Can you work these out from the model? Positions are in its coordinate system, mm. Coordinates: 2 decimals unless noted, no trailing zeros. Put each result on its own line as item: value. Start each with the question number.
from build123d import *

# Parameters (mm, degrees)
ESQUISSE1_W             = 149
ESQUISSE1_H             = 10
BOSS_EXTRU_1_DEPTH      = 3
ESQUISSE2_R             = 1.005
ESQUISSE2_W             = 5
ESQUISSE2_H             = 3
ENL_V_MAT_EXTRU_1_DEPTH = 150.365323954


with BuildPart() as part:
    # Esquisse1 → Boss.-Extru.1 (new body)
    with BuildSketch(Plane.XY):
        with Locations((74.5, 5)):
            Rectangle(ESQUISSE1_W, ESQUISSE1_H)
    extrude(amount=BOSS_EXTRU_1_DEPTH)

    # Esquisse2 → Enlèv. mat.-Extru.1 (cut, through all)
    with BuildSketch(Plane(origin=(0, 0, 0), x_dir=(-1, 0, 0), z_dir=(0, 0, -1))):
        with Locations((-3, 3)):
            Circle(ESQUISSE2_R)
        with Locations((-146, 3)):
            Circle(ESQUISSE2_R)
        with Locations((-136.5, 6.5)):
            Rectangle(ESQUISSE2_W, ESQUISSE2_H)
        with Locations((-126.5, 6.5)):
            Rectangle(ESQUISSE2_W, ESQUISSE2_H)
        with Locations((-116.5, 6.5)):
            Rectangle(ESQUISSE2_W, ESQUISSE2_H)
        with Locations((-106.5, 6.5)):
            Rectangle(ESQUISSE2_W, ESQUISSE2_H)
        with Locations((-96.5, 6.5)):
            Rectangle(ESQUISSE2_W, ESQUISSE2_H)
        with Locations((-86.5, 6.5)):
            Rectangle(ESQUISSE2_W, ESQUISSE2_H)
        with Locations((-76.5, 6.5)):
            Rectangle(ESQUISSE2_W, ESQUISSE2_H)
        with Locations((-66.5, 6.5)):
            Rectangle(ESQUISSE2_W, ESQUISSE2_H)
        with Locations((-56.5, 6.5)):
            Rectangle(ESQUISSE2_W, ESQUISSE2_H)
        with Locations((-46.5, 6.5)):
            Rectangle(ESQUISSE2_W, ESQUISSE2_H)
        with Locations((-36.5, 6.5)):
            Rectangle(ESQUISSE2_W, ESQUISSE2_H)
        with Locations((-26.5, 6.5)):
            Rectangle(ESQUISSE2_W, ESQUISSE2_H)
        with Locations((-16.5, 6.5)):
            Rectangle(ESQUISSE2_W, ESQUISSE2_H)
    extrude(amount=-ENL_V_MAT_EXTRU_1_DEPTH, mode=Mode.SUBTRACT)


solid = part.part
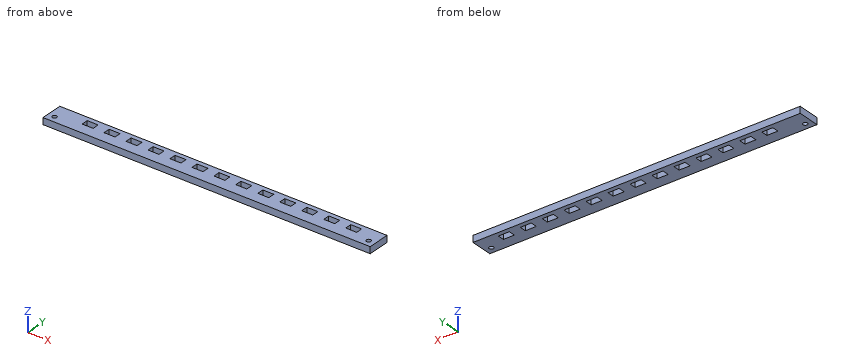
Q1. Will this pin go through, and if not, where does the flat tip stop? pin 1 (0.9 mm diameter, centred on x = 107, z = 1, fed in from -Y).
Q2. I want a section at A-A on y = 6.5. Count the separate pieces of the cut face and the enclosed holes in it, and give its area (3 significant figures).
Q3. Please list where these lines run through material, in increasing order: line 1 along Y through (x, z) = (3, 1.7) (3 decimals); line 2 along Y through (x, z) = (46, 1.8); line 3 along X through (y, z) = (2.5, 1.65). Write a range as [from, to].
Calculated:
1. pin 1: y = 0
2. separate pieces: 14
2. enclosed holes: 0
2. area: 252 mm2
3. line 1: [0, 1.995], [4.005, 10]
3. line 2: [0, 5], [8, 10]
3. line 3: [0, 2.13], [3.87, 145.13], [146.87, 149]
